Answer from the drawing. Dimensions are ordinates in mm from the lowest x, y and z of the part. A direction names the side the tool comes from. Coordinates: 2 decimals unless noted, no trailing zeros. Order: outer loops, then holes, each group sorted by start corner. A loop starts at its lowest first (then second) coordinate and runs counter-clockwise, first axis right, second up. Notation, with made-up numbers: (0.5, 57) -> (7.5, 57) arc R23 ccw to (7.5, 89) -> close; hole circle Ø4 at (-12, 51.25). An arc over 180 degrees is marked (long way). Answer in a Markdown table with one row per item.
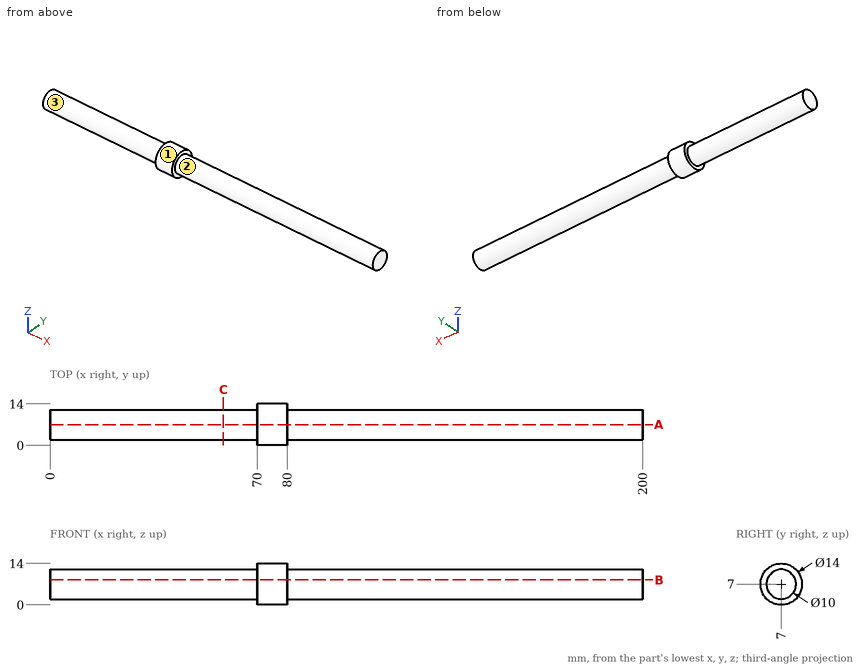
(1) Flat-ended cylindrical pins translate along their axes: pin 1 (5 mm diameter, centred on x = 135, z = 5.5, fed in from +Y); pin 2 (1 mm diameter, centred on x = 104.5, z = 10, fed in from -Y); pin 3 (1.5 mm diameter, centred on x = 156.5, y = 2, fed in from -Z). Find the tip coordinate at first contact, or state that the pin passes through.
Check values:
| item | result |
|---|---|
| pin 1 | y = 12 |
| pin 2 | y = 2.67 |
| pin 3 | z = 4.37 |
(2) A cutting plane is placed at B-B, the plane z = 8.5. Determine the outline of the cut face in (x, y).
Check values:
| item | result |
|---|---|
| outline | (0, 2.23) -> (70, 2.23) -> (70, 0.16) -> (80, 0.16) -> (80, 2.23) -> (200, 2.23) -> (200, 11.77) -> (80, 11.77) -> (80, 13.84) -> (70, 13.84) -> (70, 11.77) -> (0, 11.77) -> close |
(3) Find the intervals of material crossed by line 1 along Y through (x, z) = (164.5, 7.25); line 2 along X through (y, z) = (9.25, 11.75), in increasing order. Write a range as from..to.
Check values:
| item | result |
|---|---|
| line 1 | 2.01..11.99 |
| line 2 | 70..80 |
(4) A cutting plane is placed at C-C, the plane x = 58.5. Determine the outline of the cut face in (y, z).
Check values:
| item | result |
|---|---|
| outline | circle Ø10 at (7, 7) |
(5) A cutting plane is placed at A-A, the plane y = 7. Determine the outline of the cut face in (x, z), then the cut area to 3 significant figures.
Check values:
| item | result |
|---|---|
| outline | (0, 2) -> (70, 2) -> (70, 0) -> (80, 0) -> (80, 2) -> (200, 2) -> (200, 12) -> (80, 12) -> (80, 14) -> (70, 14) -> (70, 12) -> (0, 12) -> close |
| area | 2,040 mm² |
(6) Which of the six approach directions +Z, -Z, +X, -X, +Y, -Y give full straight-line access (tool end or side, diameter ignored) to the marked faces 1, 2 and 3?
Check values:
| item | result |
|---|---|
| face 1 | +X, -X |
| face 2 | +X |
| face 3 | -X |
